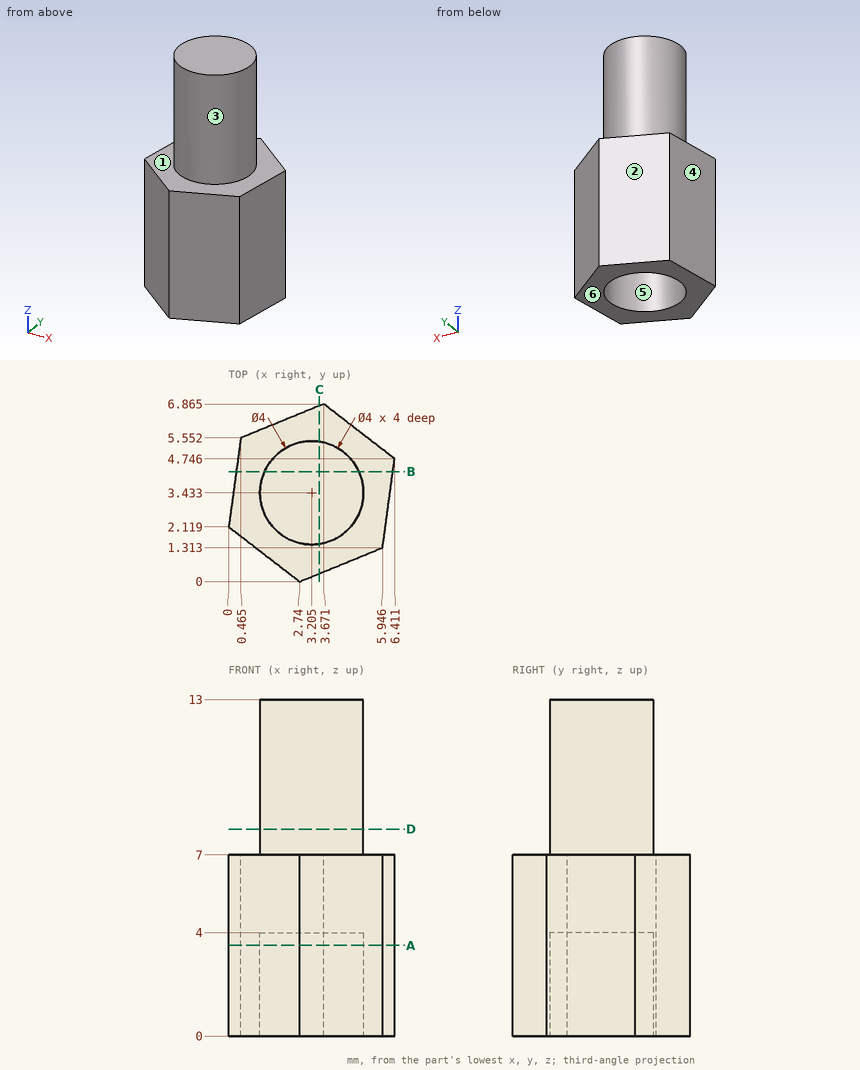
Answer from the drawing. Dimensions are ordinates in mm from the lowest x, y and z of the part. A direction names the side the tool comes from. Give positions to 0.01 mm unless a question says otherwise; leave off trailing zeros. Loops run counter-clockwise (first coordinate to the right, second up) from the corner with the lowest first, then second, coordinate; pieces in that order, holes last. Notation, with made-up numbers: (1, -0.5) - (9, -0.5) arc R13 cw to (9, 17.5) - close; hole circle Ø4 at (40, -14). An arc over 180 degrees is marked (long way). Answer as CSV lines item,"result". Start each with the question number.
Item 1: The mould has two halves that part along Y. Classify the marked faces 3, 4, 5 and 6: +Y half, -Y half, draft (parallel to the pull), parting line (faces both ways), or undercut.
Item 2: Find the intervals of material crossed by line 1 (Z direction, x = 5.5, y = 3); line 2 (Z direction, x = 4.25, y = 4); line 3 (X direction, y = 2, z = 3) (1 decimal), in increasing order. Write a range as from..to.
Item 3: A cutting plane is placed at C-C on x = 3.5. Determine the outline of the cut face in (y, z) (1 decimal).
Item 4: A cutting plane is placed at D-D on z = 8. Determine the outline of the cut face in (x, y) (1 decimal), then the cut area to 3 significant figures.
Item 5: For the marked faces 1 and 2, determine the directions among +Z, -Z, +X, -X, +Y, -Y from which every point of the face is accessible in a straight line to the end or side of a thin tool.
Item 6: A cutting plane is placed at A-A on z = 3.5. Determine the outline of the cut face in (x, y) (1 decimal).
Item 7: Each of these flat-tipped pins is pushed along its axis until it touches: pin 1 (2 mm diameter, centred on x = 3, z = 4.5, fed in from -Y); pin 2 (1.5 mm diameter, centred on x = 1, z = 11, fed in from -Y); pin 3 (1.2 mm diameter, centred on x = 2.5, y = 2.5, fed in from -Z). Where does it stop, or does it pass through?
Item 8: A cutting plane is placed at B-B on y = 4.25. Determine the outline of the cut face in (x, z).
Found:
1,face 3,"parting line"
1,face 4,"+Y half"
1,face 5,"undercut"
1,face 6,"draft"
2,line 1,"z = 0..7"
2,line 2,"z = 4..13"
2,line 3,"x = 0.2..1.8, 4.6..6"
3,outline,"(0.3, 0) - (1.5, 0) - (1.5, 4) - (5.4, 4) - (5.4, 0) - (6.8, 0) - (6.8, 7) - (5.4, 7) - (5.4, 13) - (1.5, 13) - (1.5, 7) - (0.3, 7) - close"
4,outline,"circle Ø4 at (3.2, 3.4)"
4,area,"12.6 mm^2"
5,face 1,"+Z"
5,face 2,"+Z, -Z, -X, +Y"
6,outline,"(0, 2.1) - (2.7, 0) - (5.9, 1.3) - (6.4, 4.7) - (3.7, 6.9) - (0.5, 5.6) - close; hole circle Ø4 at (3.2, 3.4)"
7,pin 1,"stops at y = 0"
7,pin 2,"stops at y = 2.06"
7,pin 3,"stops at z = 4"
8,outline,"(0.29, 0) - (1.38, 0) - (1.38, 4) - (5.03, 4) - (5.03, 0) - (6.34, 0) - (6.34, 7) - (5.03, 7) - (5.03, 13) - (1.38, 13) - (1.38, 7) - (0.29, 7) - close"
